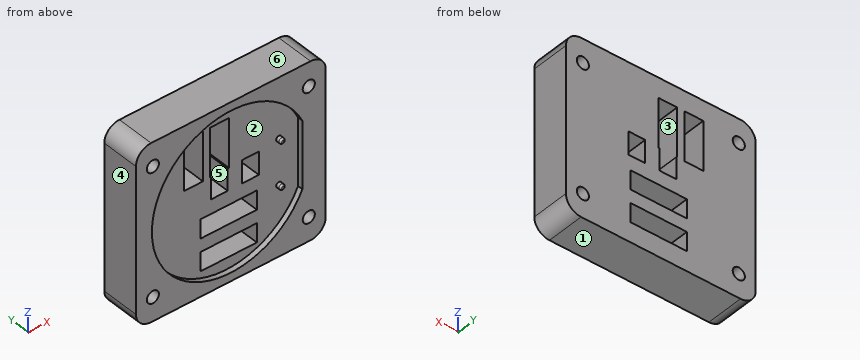
```python
from build123d import *

# Parameters (mm, degrees)
SKETCH3_W           = 31.75
SKETCH3_H           = 29.21
BOSS_EXTRUDE2_DEPTH = 6.35
CUT_EXTRUDE1_DEPTH  = 0.8636
SKETCH6_R           = 1.016
CUT_EXTRUDE3_DEPTH  = 8.89
SKETCH4_W           = 9.4234
SKETCH4_H           = 3.1496
SKETCH4_W_2         = 3.1496
SKETCH4_H_2         = 8.1534
CUT_EXTRUDE2_DEPTH  = 6.4864
SKETCH7_W           = 2.794
SKETCH7_H           = 3.81
CUT_EXTRUDE4_DEPTH  = 6.4864
FILLET1_R           = 2.54
SKETCH9_R           = 0.4445
BOSS_EXTRUDE3_DEPTH = 0.8128
FILLET2_R           = 0.254


with BuildPart() as part:
    # Sketch3 → Boss-Extrude2 (new body)
    with BuildSketch(Plane(origin=(0, 0, 0), x_dir=(1, 0, 0), z_dir=(0, 1, 0))):
        Rectangle(SKETCH3_W, SKETCH3_H)
    extrude(amount=BOSS_EXTRUDE2_DEPTH)

    # Sketch1 → Cut-Extrude1 (cut)
    with BuildSketch(Plane(origin=(0, 0, 0), x_dir=(1, 0, 0), z_dir=(0, 1, 0))):
        with BuildLine():
            Line((11.967686493, 5.588), (11.967686493, -5.588))
            ThreePointArc((11.967686493, -5.588), (-13.208, 0), (11.967686493, 5.588))
        make_face()
    extrude(amount=CUT_EXTRUDE1_DEPTH, mode=Mode.SUBTRACT)

    # Sketch6 → Cut-Extrude3 (cut)
    with BuildSketch(Plane(origin=(0, 6.35, 0), x_dir=(1, 0, 0), z_dir=(0, 1, 0))):
        with Locations((-13.0429, 10.6553)):
            Circle(SKETCH6_R)
        with Locations((13.0429, 10.6553)):
            Circle(SKETCH6_R)
        with Locations((13.0429, -10.6553)):
            Circle(SKETCH6_R)
        with Locations((-13.0429, -10.6553)):
            Circle(SKETCH6_R)
    extrude(amount=-CUT_EXTRUDE3_DEPTH, mode=Mode.SUBTRACT)

    # Sketch4 → Cut-Extrude2 (cut, through all)
    with BuildSketch(Plane.XZ.offset(-0.8636)):
        with Locations((0.3556, -9.758937639)):
            Rectangle(SKETCH4_W, SKETCH4_H)
        with Locations((-5.5245, 7.220962361)):
            Rectangle(SKETCH4_W_2, SKETCH4_H_2)
        with Locations((0.3556, -4.424937639)):
            Rectangle(SKETCH4_W, SKETCH4_H)
        with Locations((-1.1557, 7.220962361)):
            Rectangle(SKETCH4_W_2, SKETCH4_H_2)
    extrude(amount=-CUT_EXTRUDE2_DEPTH, mode=Mode.SUBTRACT)

    # Sketch7 → Cut-Extrude4 (cut, through all)
    with BuildSketch(Plane.XZ.offset(-0.8636)):
        with Locations((-1.201434663, 1.4224)):
            Rectangle(SKETCH7_W, SKETCH7_H)
        with Locations((4.005565337, 1.4224)):
            Rectangle(SKETCH7_W, SKETCH7_H)
    extrude(amount=-CUT_EXTRUDE4_DEPTH, mode=Mode.SUBTRACT)

    # Fillet1
    fillet1_edges = [part.edges().sort_by_distance(p)[0] for p in [
        (-15.875, 3.175, -14.605),
        (15.875, 3.175, -14.605),
        (15.875, 3.175, 14.605),
        (-15.875, 3.175, 14.605),
    ]]
    fillet(fillet1_edges, radius=FILLET1_R)

    # Sketch9 → Boss-Extrude3 (add)
    with BuildSketch(Plane.XZ.offset(-0.8636)):
        with Locations((8.7503, 3.7592)):
            Circle(SKETCH9_R)
        with Locations((8.7503, -3.7592)):
            Circle(SKETCH9_R)
    extrude(amount=BOSS_EXTRUDE3_DEPTH)

    # Fillet2
    fillet2_edges = [part.edges().sort_by_distance(p)[0] for p in [
        (8.3058, 0.0508, 3.7592),
        (8.3058, 0.0508, -3.7592),
    ]]
    fillet(fillet2_edges, radius=FILLET2_R)


solid = part.part
```
The listing builds one solid part. Answer for the finished solid, in the listing's coordinates (mm). Face numbers are marked on the shaded views. A direction names the side the tool comes from. Give positions to 0.01 mm unless a question says otherwise; leave off trailing zeros. Order: outer loops, then holes, each group sorted by start corner. A loop starts at its lowest first (then second) coordinate and runs counter-clockwise, first axis right, second up. Notation, with made-up numbers: (76.25, 16) -> (117.25, 16) arc R19 ccw to (117.25, 50) -> close; hole circle Ø11 at (7.5, 33.5). An arc over 180 degrees is marked (long way). Write each question's results on one line, items separated by ' | '.
Q1. The part is cut by section B-B, the plane x = -1.5. Give the vertices of the cut face in (y, z) (3 decimals).
Checked values:
outline: (0, -14.605) -> (6.35, -14.605) -> (6.35, -11.334) -> (0.864, -11.334) -> (0.864, -13.123) -> (0, -13.123) -> close; (0, 13.123) -> (0.864, 13.123) -> (0.864, 11.298) -> (6.35, 11.298) -> (6.35, 14.605) -> (0, 14.605) -> close; (0.864, -8.184) -> (6.35, -8.184) -> (6.35, -6) -> (0.864, -6) -> close; (0.864, -2.85) -> (6.35, -2.85) -> (6.35, -0.483) -> (0.864, -0.483) -> close
Q2. Determine the mould class of the marked faces 1, 2, 3 and 4 for opening direction X: pulls with the +X half, pulls with the -X half, needs draft (parallel to the pull), parting line crosses it, or undercut.
Checked values:
face 1: needs draft | face 2: undercut | face 3: undercut | face 4: pulls with the -X half
Q3. The part is cut by section C-C, the plane z = -6.5. Give the vertices of the cut face in (x, y) (3 decimals), and give its area (3 significant figures).
Checked values:
outline: (-15.875, 0) -> (-11.498, 0) -> (-11.498, 0.864) -> (11.498, 0.864) -> (11.498, 0) -> (15.875, 0) -> (15.875, 6.35) -> (-15.875, 6.35) -> close | area: 182 mm^2
Q4. Which of the six approach directions +Z, -Z, +X, -X, +Y, -Y give full straight-line access (tool end or side, diameter ignored) to the marked faces 5 and 6?
Checked values:
face 5: +Y, -Y | face 6: +Z, +X, -X, +Y, -Y
Q5. Straight lines are drawn through the part: probe 1 along X at (y, z) = (6, 2.75) (3 decimals); probe 2 along Z at (x, y) = (-13, 1) (3 decimals); probe 3 along X at (y, z) = (3.25, 3.75) (1 decimal). For each, find the intervals that lie inside material, in ascending order. Write a range as from..to.
Checked values:
probe 1: x = -15.875..-2.598, 0.196..2.609, 5.403..15.875 | probe 2: z = -14.605..-11.67, -9.64..9.64, 11.67..14.605 | probe 3: x = -15.9..-7.1, -3.9..-2.7, 0.4..15.9
Q6. The part is cut by section A-A, the plane z = 0. Give the vertices of the cut face in (x, y) (3 decimals), and give its area (3 significant figures).
Checked values:
outline: (-15.875, 0) -> (-13.208, 0) -> (-13.208, 0.864) -> (-2.598, 0.864) -> (-2.598, 6.35) -> (-15.875, 6.35) -> close; (0.196, 0.864) -> (2.609, 0.864) -> (2.609, 6.35) -> (0.196, 6.35) -> close; (5.403, 0.864) -> (11.968, 0.864) -> (11.968, 0) -> (15.875, 0) -> (15.875, 6.35) -> (5.403, 6.35) -> close | area: 149 mm^2
Q7. Each of these flat-tipped pins is pushed along its axis until it touches: P1, Ø8, axis at x = 9, z = 7.5, coming from the -Y side; P2, Ø3, axis at x = 0, z = -1, coming from the -Y side. Where does it stop, or does it pass through?
Checked values:
P1: stops at y = 0 | P2: stops at y = 0.86
